Read the model definition and answer for the solid it produces. Units are mm, in the model's axes. Face numbers are marked on the shaded views. A direction names the side the tool comes from. Give positions to 0.01 mm unless a question says otherwise; leave off trailing zeros. Write each loop counter-clockwise with the first axis right and the second up, starting at its lowest first coordinate (ties: lowest second). Pieces come first, ordered by that corner, then holes.
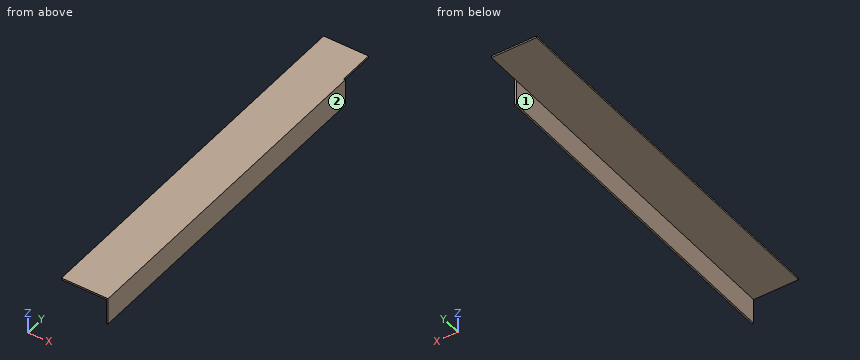
```python
from build123d import *

# Parameters (mm, degrees)
F1_DEPTH = 4.7625
F2_W     = 965.2
F2_H     = 76.2
F3_DEPTH = 4.7625


with BuildPart() as f1:
    # F0 (on Top) → F1 (new body)
    with BuildSketch(Plane.XY):
        Polygon((63.5, -381), (63.5, 533.4), (-63.5, 533.4), (-63.5, -533.4), (63.5, -533.4), align=None)
    extrude(amount=F1_DEPTH)

    # F2 (on face) → F3 (join)
    with BuildSketch(Plane.YZ.offset(63.5)):
        with Locations((-50.8, -33.3375)):
            Rectangle(F2_W, F2_H)
    extrude(amount=F3_DEPTH)


solid = f1.part
```
Item 1: Find the intervals of material crossed by line 1 along Z through (x, y) = (-12, -246.5); line 2 along X through (y, z) = (28, -60), in increasing order.
Result set:
line 1: z = 0 to 4.76
line 2: x = 63.5 to 68.26
Item 2: Each of these flat-tipped pins is pushed along its axis until it touches: pin 1 Ø10 at (y, z) = (-307, -56.5) entering from -X; pin 2 Ø1.4 at (x, z) = (65, -47.5) entering from +Y; pin 3 Ø10 at (x, y) = (17, -132) entering from -Z. Where does it stop, or does it pass through?
Result set:
pin 1: stops at x = 63.5
pin 2: stops at y = 431.8
pin 3: stops at z = 0
Item 3: Section C-C (x = -28) is taken. Write down the section's boundary in (y, z).
Result set:
outline: (-533.4, 0) - (533.4, 0) - (533.4, 4.76) - (-533.4, 4.76) - close
Item 4: Section A-A (y = 96) is taken. Write down the section's boundary in (x, z), and give its area (3 significant figures).
Result set:
outline: (-63.5, 0) - (63.5, 0) - (63.5, -71.44) - (68.26, -71.44) - (68.26, 4.76) - (-63.5, 4.76) - close
area: 968 mm2
Item 5: Section B-B (z = -12) is taken. Write down the section's boundary in (x, y), and give its area (3 significant figures).
Result set:
outline: (63.5, -533.4) - (68.26, -533.4) - (68.26, 431.8) - (63.5, 431.8) - close
area: 4,600 mm2
Item 6: Which of the six approach directions +Z, -Z, +X, -X, +Y, -Y give full straight-line access (tool end or side, diameter ignored) to the marked faces 1 and 2?
Result set:
face 1: -Z, -X, +Y, -Y
face 2: +Z, -Z, +X, +Y, -Y
